from build123d import *

# Parameters (mm, degrees)
BOSS_EXTRUDE1_DEPTH = 6.35
CUT_EXTRUDE1_DEPTH  = 145.787309477
SKETCH3_W           = 73.915341148
SKETCH3_H           = 6.35
BOSS_EXTRUDE2_DEPTH = 7.62
CUT_EXTRUDE2_DEPTH  = 145.787309477
FILLET1_R           = 3.175
SKETCH5_R           = 2.54
CUT_EXTRUDE3_DEPTH  = 113.806666284


with BuildPart() as part:
    # Sketch1 → Boss-Extrude1 (new body)
    with BuildSketch(Plane(origin=(0, 0, 0), x_dir=(1, 0, 0), z_dir=(0, 1, 0))):
        Polygon((0, 0), (34.173489324, 95.680366991), (108.087489324, 96.125632051), (73.914, 0.44526506), align=None)
    extrude(amount=BOSS_EXTRUDE1_DEPTH)

    # Sketch2 → Cut-Extrude1 (cut, through all)
    with BuildSketch(Plane(origin=(0, 6.35, 0), x_dir=(1, 0, 0), z_dir=(0, 1, 0))):
        with BuildLine():
            ThreePointArc((55.234228554, 47.840183495), (53.964228554, 49.110183495), (52.694228554, 47.840183495))
            Line((52.694228554, 47.840183495), (55.234228554, 47.840183495))
        make_face()
        with BuildLine():
            Line((55.234228554, 47.840183495), (52.694228554, 47.840183495))
            ThreePointArc((52.694228554, 47.840183495), (53.964228554, 46.570183495), (55.234228554, 47.840183495))
        make_face()
    extrude(amount=-CUT_EXTRUDE1_DEPTH, mode=Mode.SUBTRACT)

    # Sketch3 → Boss-Extrude2 (add)
    with BuildSketch(Plane(origin=(0, 0, 0), x_dir=(0.9999818556252084, 0, -0.00602398708207968), z_dir=(0.00602398708207968, 0, 0.9999818556252085))):
        with Locations((36.957670574, 3.175)):
            Rectangle(SKETCH3_W, SKETCH3_H)
    extrude(amount=BOSS_EXTRUDE2_DEPTH)

    # Sketch4 → Cut-Extrude2 (cut, through all)
    with BuildSketch(Plane(origin=(0, 6.35, 0), x_dir=(1, 0, 0), z_dir=(0, 1, 0))):
        Polygon((15.256454596, 0.091906353), (0, 0), (0.045902782, -7.61986174), (15.256454596, -7.52823191), align=None)
        Polygon((44.594795755, 0.268643348), (29.354795755, 0.176836119), (29.354795755, -7.443302144), (44.594795755, -7.351494915), align=None)
        Polygon((73.914, 0.44526506), (58.693136915, 0.353573114), (58.693136915, -7.266565149), (73.959902782, -7.17459668), align=None)
    extrude(amount=-CUT_EXTRUDE2_DEPTH, mode=Mode.SUBTRACT)

    # Fillet1
    fillet1_edges = [part.edges().sort_by_distance(p)[0] for p in [
        (51.643966335, 0, 7.309030032),
        (51.643966335, 6.35, 7.309030032),
        (22.305625176, 0, 7.485767027),
        (22.305625176, 6.35, 7.485767027),
    ]]
    fillet(fillet1_edges, radius=FILLET1_R - 0.0001)  # a hair under: the kernel refuses the full size

    # Sketch5 → Cut-Extrude3 (cut, through all)
    with BuildSketch(Plane(origin=(58.693136915, 0, 0), x_dir=(0, 0, -1), z_dir=(1, 0, 0))):
        with Locations((-4.091507539, 3.175)):
            Circle(SKETCH5_R)
    extrude(amount=-CUT_EXTRUDE3_DEPTH, mode=Mode.SUBTRACT)


solid = part.part
Work out the finished part from the listing and answer in its coordinate system (mm). A direction names the side the tool comes from. Round coordinates to 2 decimals unless told otherwise and drop trailing zeros. Write each loop counter-clockwise with the first axis right and the second up, starting at its lowest first coordinate (ties: lowest second). Pieces come first, ordered by that corner, then holes.
1) A tool of negligible diameter and unlimited length cuts with its end or side. For faces 5 (the cylindrical face through (51.7, 5.4, 6.4)), 6 (the cylindrical face through (51.747, 0.905, 6.354)), from which of +Z, -Z, +X, -X, +Y, -Y can it reach the whole face along a straight path? Write none if from no direction.
2) A cutting plane is placed at A-A (y = 4.75). Give the vertices of the cut face in (x, z), plus the area to 3 significant figures.
3) A cutting plane is placed at B-B (x = 89). Give the vertices of the cut face in (y, z), plus the area to 3 significant figures.
4) A cutting plane is placed at C-C (z = -3). Give the vertices of the cut face in (x, y), plus the area to 3 significant figures.
5) The mould has two halves that part along X. Classify faces 1 (the flat face through (29.355, 5, 2)), 2 (the cylindrical face through (22.4, 1.63, 6.11)), 3 (the flat face through (58.693, 3, 1)), 4 (the flat face through (16.848, 3.131, -47.17)): pulls with the +X half, pulls with the -X half, needs draft (parallel to the pull), parting line crosses it, or undercut.
6) Straight lines are drawn through the part: line 1 (Z direction, x = 57, y = 1.5); line 2 (X direction, y = 5.5, z = -65); line 3 (Z direction, x = 73, y = 1). For each, find the intervals that lie inside material, in ascending order.
7) Given pin 1 Ø1.9 at (y, z) = (2, 2.5) entering from +X; pin 2 Ø1 at (y, z) = (3, -29) entering from +X; pin 3 Ø1 at (x, y) = (74, 2) entering from +Z, each flat-ended and moving along its own axis, determine where each tip first touches the part or whether it passes through.
Completed:
1. face 5: +Z, +X, +Y
1. face 6: +Z, +X, -Y
2. outline: (0, 0) - (34.17, -95.68) - (108.09, -96.13) - (73.91, -0.45) - (58.69, -0.35) - (58.69, 2.1) - (44.59, 2.1) - (44.59, -0.27) - (29.35, -0.18) - (29.35, 2.1) - (15.26, 2.1) - (15.26, -0.09) - close; (15.26, 6.08) - (29.35, 6.08) - (29.35, 7.03) - (15.26, 7.11) - close; (44.59, 6.08) - (58.69, 6.08) - (58.69, 6.85) - (44.59, 6.93) - close; hole circle Ø2.54 at (53.96, -47.84)
2. area: 7,140 mm2
3. outline: (0, -96.01) - (6.35, -96.01) - (6.35, -42.68) - (0, -42.68) - close
3. area: 339 mm2
4. outline: (1.07, 0) - (74.83, 0) - (74.83, 6.35) - (1.07, 6.35) - close
4. area: 468 mm2
5. face 1: undercut
5. face 2: needs draft
5. face 3: pulls with the +X half
5. face 4: pulls with the -X half
6. line 1: z = -95.82 to 2.18, 6 to 6.8
6. line 2: x = 23.22 to 96.97
6. line 3: z = -95.91 to -0.44
7. pin 1: stops at x = 58.69
7. pin 2: stops at x = 84.29
7. pin 3: stops at z = -0.44
